from build123d import *

# Parameters (mm, degrees)
SKETCH_1_R          = 30
SKETCH_1_R_2        = 10.1
EXTRUDE_1_DEPTH     = 5
EXTRUDE_2_DEPTH     = 27
SKETCH_3_R          = 3.1
CUT_EXTRUDE_1_DEPTH = 3
SKETCH_4_R          = 1.6
CUT_EXTRUDE_2_DEPTH = 52.961524227
FILLET_1_R          = 1


with BuildPart() as part:
    # 草图1 → 凸台-拉伸1 (new body)
    with BuildSketch(Plane(origin=(0, 0, 0), x_dir=(0, 0, -1), z_dir=(1, 0, 0))):
        Circle(SKETCH_1_R)
        Circle(SKETCH_1_R_2, mode=Mode.SUBTRACT)
    extrude(amount=EXTRUDE_1_DEPTH)

    # 草图2 → 凸台-拉伸2 (add)
    with BuildSketch(Plane.ZY):
        with BuildLine():
            Line((-3, 20.784609691), (-3, 17.748239349))
            ThreePointArc((-3, 17.748239349), (-15.588457268, 9), (-16.870426149, -6.276043463))
            Line((-16.870426149, -6.276043463), (-19.5, -7.794228634))
            ThreePointArc((-19.5, -7.794228634), (-18.186533479, 10.5), (-3, 20.784609691))
        make_face()
        with BuildLine():
            Line((3, 20.784609691), (3, 17.748239349))
            ThreePointArc((3, 17.748239349), (15.588457268, 9), (16.870426149, -6.276043463))
            Line((16.870426149, -6.276043463), (19.5, -7.794228634))
            ThreePointArc((19.5, -7.794228634), (18.186533479, 10.5), (3, 20.784609691))
        make_face()
        with BuildLine():
            Line((16.5, -12.990381057), (13.870426149, -11.472195886))
            ThreePointArc((13.870426149, -11.472195886), (0, -18), (-13.870426149, -11.472195886))
            Line((-13.870426149, -11.472195886), (-16.5, -12.990381057))
            ThreePointArc((-16.5, -12.990381057), (0, -21), (16.5, -12.990381057))
        make_face()
    extrude(amount=EXTRUDE_2_DEPTH)

    # 草图3 → 切除-拉伸1 (cut)
    with BuildSketch(Plane.ZY):
        with Locations((0, 15)):
            Circle(SKETCH_3_R)
        with Locations((12.990381057, -7.5)):
            Circle(SKETCH_3_R)
        with Locations((-12.990381057, -7.5)):
            Circle(SKETCH_3_R)
    extrude(amount=-CUT_EXTRUDE_1_DEPTH, mode=Mode.SUBTRACT)

    # 草图4 → 切除-拉伸2 (cut, through all)
    with BuildSketch(Plane.ZY.offset(-3)):
        with Locations((0, 15)):
            Circle(SKETCH_4_R)
        with Locations((12.990381057, -7.5)):
            Circle(SKETCH_4_R)
        with Locations((-12.990381057, -7.5)):
            Circle(SKETCH_4_R)
    extrude(amount=-CUT_EXTRUDE_2_DEPTH, mode=Mode.SUBTRACT)

    # 圆角1
    fillet_1_edges = [part.edges().sort_by_distance(p)[0] for p in [
        (0, 10.5, -18.186533479),
        (-13.5, 20.784609691, -3),
        (0, -7.035136049, -18.185213074),
        (-13.5, -7.794228634, -19.5),
        (0, 9, -15.588457268),
        (-13.5, -6.276043463, -16.870426149),
        (0, 19.26642452, -3),
        (-13.5, 17.748239349, -3),
        (-27, -7.035136049, -18.185213074),
        (-27, 19.26642452, -3),
        (0, -21, 0),
        (-13.5, -12.990381057, -16.5),
        (0, -12.231288471, 15.185213074),
        (-13.5, -12.990381057, 16.5),
        (0, -18, 0),
        (-13.5, -11.472195886, 13.870426149),
        (0, -12.231288471, -15.185213074),
        (-13.5, -11.472195886, -13.870426149),
        (-27, -12.231288471, 15.185213074),
        (-27, -12.231288471, -15.185213074),
        (0, 10.5, 18.186533479),
        (-13.5, -7.794228634, 19.5),
        (0, 19.26642452, 3),
        (-13.5, 20.784609691, 3),
        (0, 9, 15.588457268),
        (-13.5, 17.748239349, 3),
        (0, -7.035136049, 18.185213074),
        (-13.5, -6.276043463, 16.870426149),
        (-27, 19.26642452, 3),
        (-27, -7.035136049, 18.185213074),
    ]]
    fillet(fillet_1_edges, radius=FILLET_1_R)


solid = part.part
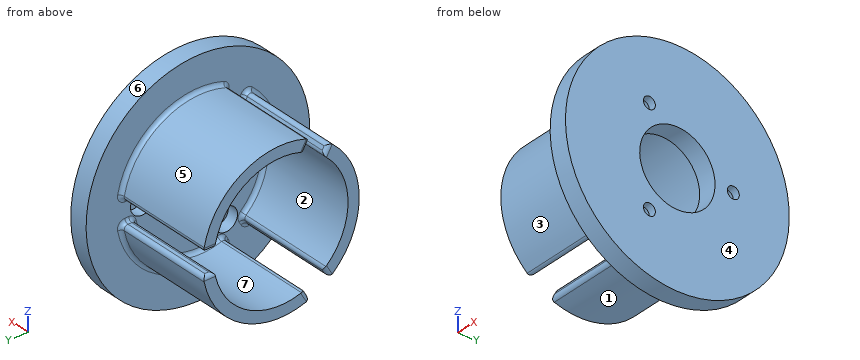
Design review of the part built by this model. Coordinates are the model's own, in mm. Face numbers are marked on the shaded views. A direction names the side the tool comes from. Give positions to 0.01 mm unless a question says otherwise; leave off trailing zeros. Loops run counter-clockwise (first coordinate to the right, second up) from the corner with the lowest first, then second, coordinate; pieces in that order, holes last. Notation, with made-up numbers: M 65.5,-21 L 87.5,-21 A10 ccw 87.5,-7 Z; hole C 70,-16 d6. An arc over 180 degrees is marked long. Answer as a JSON object with one key per item and string values.
Item 1: We need section C-C (y = -23). State the section outline as (x, z) points, and give its area (3 significant figures).
Output values:
{"outline": "M 0,-19.26 L 5,-19.26 L 5,19.26 L 0,19.26 Z", "area": "193 mm2"}
Item 2: Machinability: for the marked faces 5, 6 and 7, which of the approach directions +Z, -Z, +X, -X, +Y, -Y give a long, thin tool a straight path to every point of the face, cutting with its end or side? Answer none if there is none.
Output values:
{"face 5": "+Z, -X", "face 6": "+X, -X", "face 7": "-X"}
Item 3: We need section D-D (z = 25.5). State the section outline as (x, y) points, and give its area (3 significant figures).
Output values:
{"outline": "M 0,-15.8 L 5,-15.8 L 5,15.8 L 0,15.8 Z", "area": "158 mm2"}
Item 4: We need section B-B (x = -9). State the section outline as (y, z) points, and give its area (3 significant figures).
Output values:
{"outline": "M -13.93,-15.72 A1 ccw -12.4,-15.47 L -11.89,-14.59 A1 ccw -12.08,-13.34 A18 cw -12.08,13.34 A1 ccw -11.89,14.59 L -12.4,15.47 A1 ccw -13.93,15.72 A21 ccw Z; M -7.2,-18.47 A1 ccw -6.65,-19.92 A21 ccw 20.58,-4.2 A1 ccw 19.6,-3 L 18.57,-3 A1 ccw 17.6,-3.79 A18 cw -5.52,-17.13 A1 ccw -6.69,-17.59 Z; M -7.2,18.47 L -6.69,17.59 A1 ccw -5.52,17.13 A18 cw 17.6,3.79 A1 ccw 18.57,3 L 19.6,3 A1 ccw 20.58,4.2 A21 ccw -6.65,19.92 A1 ccw Z", "area": "311 mm2"}
Item 5: For P1, Ø5, axis at x = -20, z = 3.5, coming from the +Y side; P2, Ø4, axis at x = -22.5, y = 1.5, coming from the +Z side; P3, Ø1, axis at y = 21.5, z = 6.5, coming from the -X side; P4, Ø3, axis at x = -12.5, y = -23.5, coming from the +Z side, all flat-tipped, find the tip position at first contact; note any pin that passes through.
Output values:
{"P1": "stops at y = 20.6", "P2": "stops at z = 21", "P3": "stops at x = 0", "P4": "passes through"}
Item 6: Wall thickness on line 1 along Y through (x, z) = (2, 0); line 2 along Y through (x, z) = (3.7, 0); line 3 along X through (y, z) = (-24, 3): over which ranges is each line inside the solid? List them lowest first.
Output values:
{"line 1": "y = -30 to -10.1, 10.1 to 11.9, 18.1 to 30", "line 2": "y = -30 to -10.1, 10.1 to 13.4, 16.6 to 30", "line 3": "x = 0 to 5"}
Item 7: We need section A-A (z = 0). State the section outline as (x, y) points.
Output values:
{"outline": "M -27,-21 L -1,-21 A1 cw 0,-22 L 0,-30 L 5,-30 L 5,-10.1 L 0,-10.1 L 0,-17 A1 cw -1,-18 L -27,-18 Z; M 0,10.1 L 5,10.1 L 5,13.4 L 3,13.4 L 3,11.9 L 0,11.9 Z; M 0,18.1 L 3,18.1 L 3,16.6 L 5,16.6 L 5,30 L 0,30 Z"}
Item 8: Mouldability with a two-part tool opening along Y and no side actions: class the marked faces 1, 2, 3 and 4 as pulls with the +Y half, pulls with the -Y half, needs draft (parallel to the pull), parting line crosses it, or undercut.
Output values:
{"face 1": "parting line crosses it", "face 2": "undercut", "face 3": "pulls with the -Y half", "face 4": "needs draft"}
